```python
from build123d import *

# Parameters (mm, degrees)
SKETCH_1_W          = 74.4
SKETCH_1_H          = 42.9
EXTRUDE_1_DEPTH     = 3
SKETCH_2_W          = 61.56
SKETCH_2_H          = 44.02
EXTRUDE_2_DEPTH     = 3
SKETCH_3_W          = 48.96
SKETCH_3_H          = 36.72
CUT_EXTRUDE_2_DEPTH = 0.5


with BuildPart() as part:
    # 草图1 → 凸台-拉伸1 (new body)
    with BuildSketch(Plane.XY):
        Rectangle(SKETCH_1_W, SKETCH_1_H)
    extrude(amount=EXTRUDE_1_DEPTH)

    # 草图2 → 凸台-拉伸2 (add)
    with BuildSketch(Plane.XY.offset(3)):
        Rectangle(SKETCH_2_W, SKETCH_2_H)
    extrude(amount=-EXTRUDE_2_DEPTH)

    # 草图3 → 切除-拉伸2 (cut)
    with BuildSketch(Plane.XY.offset(3)):
        Rectangle(SKETCH_3_W, SKETCH_3_H)
    extrude(amount=-CUT_EXTRUDE_2_DEPTH, mode=Mode.SUBTRACT)


solid = part.part
```
Model file for the job. Use its own axes, mm. A direction names the side the tool comes from. Give positions to 0.01 mm unless a question says otherwise; leave off trailing zeros. Loops run counter-clockwise (first coordinate to the right, second up) from the corner with the lowest first, then second, coordinate; pieces in that order, holes last. Notation, with made-up numbers: (21.25, 32.25) -> (40.25, 32.25) arc R17 cw to (40.25, 41.25) -> close; hole circle Ø8 at (75.5, 44.5). An arc over 180 degrees is marked (long way). Use CSV: the item, a comma, the result in double quotes. Start each with the question number.
1) Mould opens along X. For faces 5 (the flat face through (37.2, 0, 1)), 6 (the flat face through (0, 0, 2.5)), 7 (the flat face through (34, -21.45, 1)) say: released by +X, released by -X, zero draft, split by the parting line, or undercut.
2) Slice it at A-A on y = -8. Give the cut face in (x, z).
3) Slice it at B-B on x = 9.5. Give the cut face in (y, z).
4) Tool access for faces 1 (the flat face through (34, 21.45, 1)), 2 (the flat face through (-34, -21.45, 1)), 3 (the flat face through (-34, 21.45, 1)), 4 (the flat face through (-37.2, 0, 1)): list every direction of +Z, -Z, +X, -X, +Y, -Y with a clear straight run to the whole face (end or side of a thin tool).
5) Flat gauge pins, fed straight in: pin 1 Ø8 at (x, y) = (10.5, -4.5) entering from +Z; pin 2 Ø1.5 at (x, z) = (-33.5, 2) entering from +Y; pin 3 Ø0.6 at (y, z) = (22, 1) entering from -X. Where does each tip first touch, or does it go through?
6) Wall check: line 1 (Y direction, x = -21.5, z = 2.65); line 2 (Z direction, x = 5.5, y = 17); line 3 (X direction, y = 15, z = 2.75). Give the ranges that are in metal, low to high.
Computed values:
1,face 5,"released by +X"
1,face 6,"undercut"
1,face 7,"zero draft"
2,outline,"(-37.2, 0) -> (37.2, 0) -> (37.2, 3) -> (24.48, 3) -> (24.48, 2.5) -> (-24.48, 2.5) -> (-24.48, 3) -> (-37.2, 3) -> close"
3,outline,"(-22.01, 0) -> (22.01, 0) -> (22.01, 3) -> (18.36, 3) -> (18.36, 2.5) -> (-18.36, 2.5) -> (-18.36, 3) -> (-22.01, 3) -> close"
4,face 1,"+Z, -Z, +X, +Y"
4,face 2,"+Z, -Z, -X, -Y"
4,face 3,"+Z, -Z, -X, +Y"
4,face 4,"+Z, -Z, -X, +Y, -Y"
5,pin 1,"stops at z = 2.5"
5,pin 2,"stops at y = 21.45"
5,pin 3,"stops at x = -30.78"
6,line 1,"y = -22.01 to -18.36, 18.36 to 22.01"
6,line 2,"z = 0 to 2.5"
6,line 3,"x = -37.2 to -24.48, 24.48 to 37.2"
